from build123d import *

# Parameters (mm, degrees)
F0_R     = 63.5
F1_DEPTH = 19.05
F2_R     = 6.35
F3_DEPTH = 6.35
F4_SIZE  = 12.7


with BuildPart() as f1:
    # F0 (on Top) → F1 (new body)
    with BuildSketch(Plane.XY):
        with Locations((0, -4.811709)):
            Circle(F0_R)
    extrude(amount=F1_DEPTH)

    # F2 (on face) → F3 (join)
    with BuildSketch(Plane(origin=(0, 0, 0), x_dir=(1, 0, 0), z_dir=(0, 0, -1))):
        Circle(F2_R)
    extrude(amount=F3_DEPTH)

    # F4
    f4_edges = [f1.edges().sort_by_distance(p)[0] for p in [
        (-63.5, -4.811709, 19.05),
    ]]
    chamfer(f4_edges, length=F4_SIZE)


solid = f1.part
Build history of the part. All positions in model axes, mm. A direction names the side the tool comes from. Coordinates: 2 decimals unless noted, no trailing zeros. Write each loop counter-clockwise with the first axis right and the second up, starting at its lowest first coordinate (ties: lowest second). Pieces come first, ordered by that corner, then holes.
(1) Cut at C-C on z = 12.5. List the corners of the cut face in (x, y), and give its area (3 significant figures).
(2) Cut at A-A on x = 0. List the corners of the cut face in (y, z).
(3) 3-axis set-ups, long thin cutter, end or side, ignore diameter. For faces 1 (the cylindrical face through (-1.38, 6.2, -3.13)), 2 (the cylindrical face through (-13.77, -66.8, 3.13)): which of +Z, -Z, +X, -X, +Y, -Y reach the whole face in a straight line?
(4) Pin check, flat tips, straight feed: pin 1 Ø2 at (y, z) = (13, 8) entering from +X; pin 2 Ø10 at (x, y) = (-49.5, -33) entering from +Z; pin 3 Ø12 at (y, z) = (-41, 16) entering from +X. Stop position of each tip, or through.
(5) Drill centre lines: line 1 (Z direction, x = 22, y = -0.5); line 2 (Y direction, x = -15, z = 14.25); line 3 (Y direction, x = -12, z = 11.75). Where is each one in solid material? Low to high.
(6) Cut at B-B on z = -3.5. List the corners of the cut face in (x, y), and give its area (3 significant figures).
Working result:
1. outline: circle Ø114.7 at (0, -4.81)
1. area: 10,300 mm2
2. outline: (-68.31, 0) - (-6.35, 0) - (-6.35, -6.35) - (6.35, -6.35) - (6.35, 0) - (58.69, 0) - (58.69, 6.35) - (45.99, 19.05) - (-55.61, 19.05) - (-68.31, 6.35) - close
3. face 1: -Z
3. face 2: +Z, -Z
4. pin 1: stops at x = 60.31
4. pin 2: stops at z = 17.89
4. pin 3: stops at x = 48.84
5. line 1: z = 0 to 19.05
5. line 2: y = -58.35 to 48.73
5. line 3: y = -61.66 to 52.04
6. outline: circle Ø12.7 at (0, 0)
6. area: 127 mm2
